Design review of the part shown in the three views and the two pictorial views. Dimensions are in mm from the part's minimum x, y and z. A direction names the side the tool comes from. Give positions to 0.01 mm unless a question says otherwise; leave off trailing zeros. Loops run counter-clockwise (first coordinate to the right, second up) from the corner with the lowest first, then second, coordinate; pieces in that order, holes last. Notation, with made-up numbers: (70.5, 12.5) -> (91.5, 12.5) arc R30 ccw to (91.5, 50.5) -> close; hole circle Ø2 at (14.5, -16). An arc over 180 degrees is marked (long way). Answer as CSV lines item,"result".
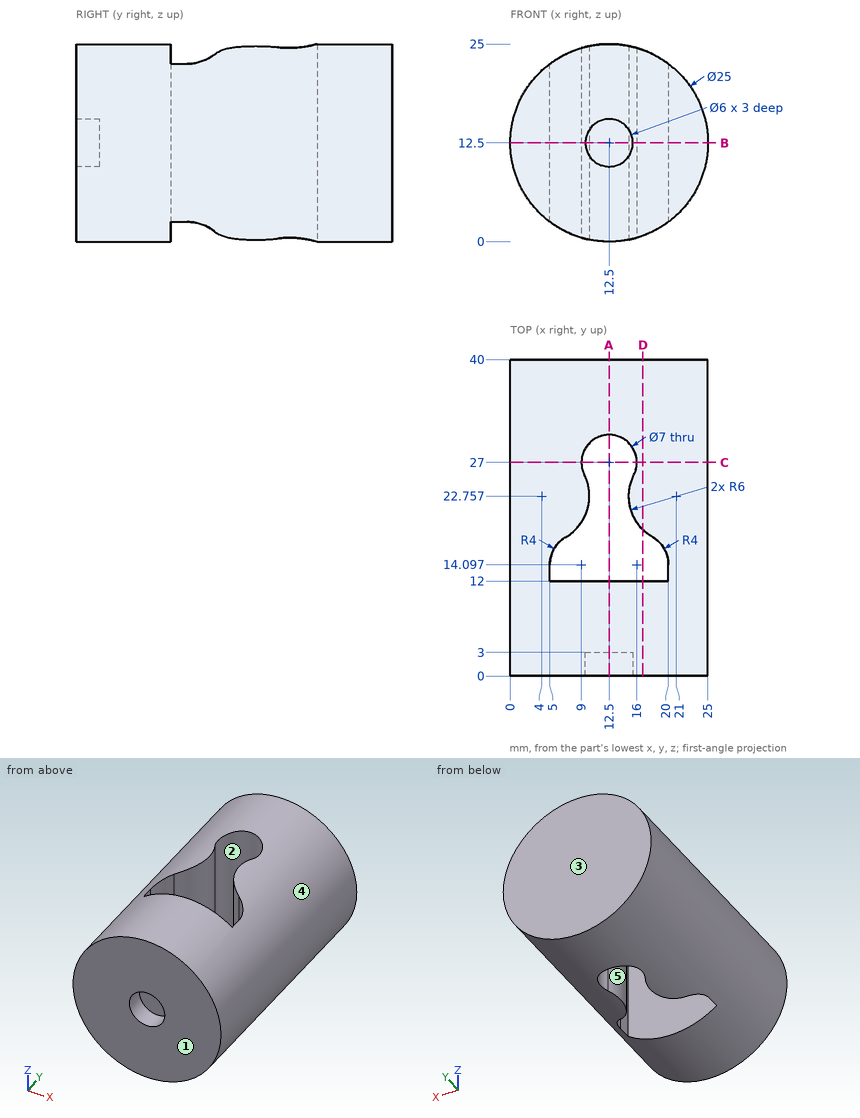
Q1. For the marked faces 4 and 5, list the 3-axis set-ups (+Z, -Z, +X, -X, +Y, -Y) from which the entire face can be reached by the end or side of a thin tool; tool diameter is ignored.
Filled sheet:
face 4,"+Y, -Y"
face 5,"+Z, -Z"
Q2. We need section B-B, the plane z = 12.5. State the section outline as (x, y) points.
Filled sheet:
outline,"(0, 0) -> (9.5, 0) -> (9.5, 3) -> (15.5, 3) -> (15.5, 0) -> (25, 0) -> (25, 40) -> (0, 40) -> close; hole (5, 12) -> (20, 12) -> (20, 14.1) arc R4 ccw to (18, 17.56) arc R6 cw to (15.63, 25.44) arc R3.5 ccw (long way) to (9.37, 25.44) arc R6 cw to (7, 17.56) arc R4 ccw to (5, 14.1) -> close"
Q3. To check wall thickness, follow probe 1 along Y at (x, z) = (12.5, 11.25); probe 2 along Y at (x, z) = (12.25, 9); probe 3 along X at (y, z) = (27, 12.75). State the ranges of each line that lie inside material, in increasing order. Write a range as from..to.
Filled sheet:
probe 1,"y = 3..12, 30.5..40"
probe 2,"y = 0..12, 30.49..40"
probe 3,"x = 0..9, 16..25"
Q4. We need section D-D, the plane x = 16.75. State the section outline as (y, z) points (1 decimal).
Filled sheet:
outline,"(0, 0.7) -> (12, 0.7) -> (12, 24.3) -> (0, 24.3) -> close; (18.5, 0.7) -> (40, 0.7) -> (40, 24.3) -> (18.5, 24.3) -> close"
Q5. We need section C-C, the plane y = 27. State the section outline as (x, z) points.
Filled sheet:
outline,"(9, 0.5) -> (9, 24.5) arc R12.5 ccw to start; (16, 0.5) arc R12.5 ccw to (16, 24.5) -> close"
Q6. Clearance check with flat-ended pins moving along their axes: pin 1 Ø2 at (x, y) = (17.5, 14.5) entering from -Z; pin 2 Ø6 at (y, z) = (33, 7.5) entering from +X; pin 3 Ø5 at (x, y) = (4.5, 11.5) entering from +Z (1 decimal); pin 4 Ø10 at (y, z) = (20.5, 21.5) entering from -X. State where each tip first meets the part, or that it passes through.
Filled sheet:
pin 1,"passes through"
pin 2,"stops at x = 24.84"
pin 3,"stops at z = 23.7"
pin 4,"stops at x = 0.66"
Q7. We need section A-A, the plane x = 12.5. State the section outline as (y, z) points.
Filled sheet:
outline,"(0, 0) -> (12, 0) -> (12, 25) -> (0, 25) -> (0, 15.5) -> (3, 15.5) -> (3, 9.5) -> (0, 9.5) -> close; (30.5, 0) -> (40, 0) -> (40, 25) -> (30.5, 25) -> close"
Q8. The part is to be moulded in two halves that separate along Y. For the marked faces 1, 2 and 3, say which applies: pulls with the +Y half, pulls with the -Y half, needs draft (parallel to the pull), parting line crosses it, or undercut.
Filled sheet:
face 1,"pulls with the -Y half"
face 2,"undercut"
face 3,"pulls with the +Y half"
